Geometry check sheet. Reference: drawing and pictorial views, mm from the part's lowest x, y, z. Coordinates: 2 decimals unless noted, no trailing zeros. Loops run counter-clockwise (first coordinate to the right, second up) from the corner with the lowest first, then second, coordinate; pieces in that order, holes last.
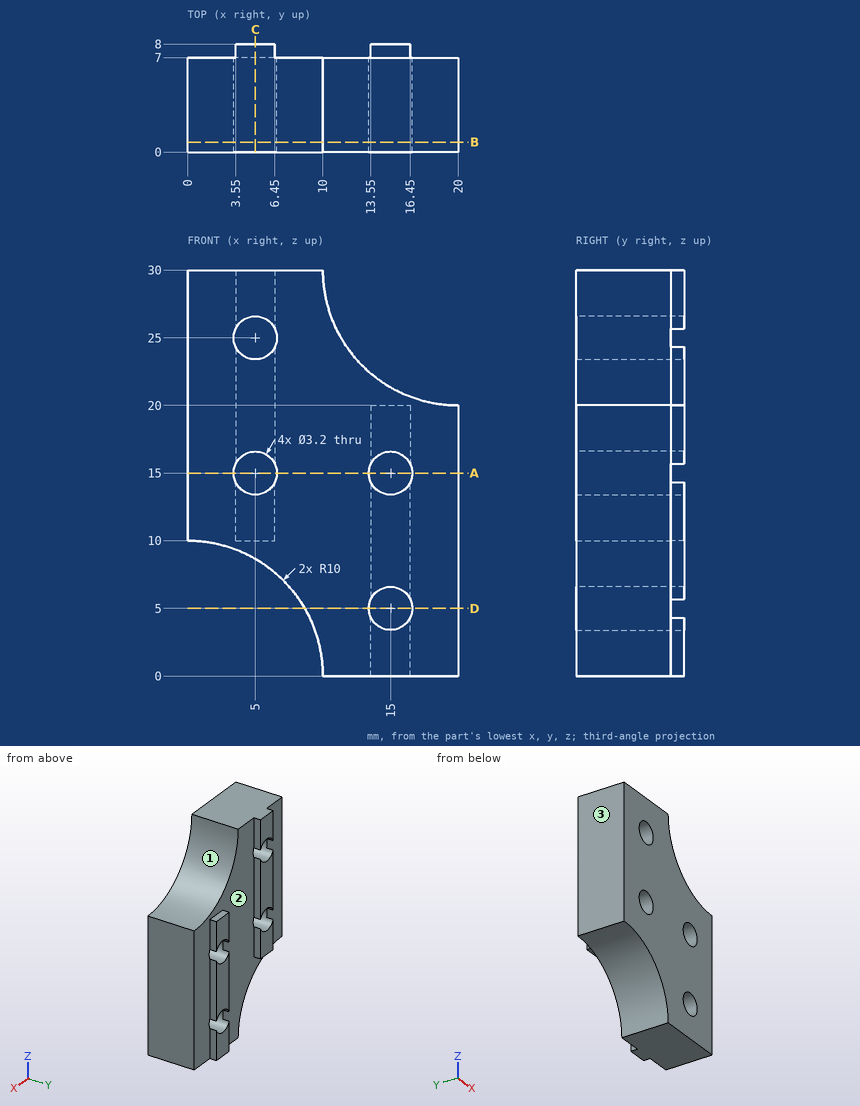
1) Depth check by flat-ended pin: pin 1 (0.8 mm diameter, centred on y = 7.5, z = 12.5, fed in from -X); pin 2 (0.8 mm diameter, centred on x = 5.5, y = 7.5, fed in from -Z); pin 3 (0.8 mm diameter, centred on y = 7.5, z = 17, fed in from +X). Enter the tip coordinate at first touch or a pass-through.
Data:
pin 1: stops at x = 3.55
pin 2: stops at z = 10
pin 3: stops at x = 16.45
2) Mould release check, pull along X, two halves, no side actions. Record for the marked faces 1, 2 and 3: +X half, -X half, draft (parallel to the pull), parting line (faces both ways), or undercut.
Data:
face 1: +X half
face 2: undercut
face 3: -X half
3) Section check C-C on x = 5. Record the cut outline in (y, z), and give its area (3 significant figures).
Data:
outline: (0, 8.66) - (7, 8.66) - (7, 10) - (8, 10) - (8, 13.4) - (0, 13.4) - close; (0, 16.6) - (8, 16.6) - (8, 23.4) - (0, 23.4) - close; (0, 26.6) - (8, 26.6) - (8, 30) - (0, 30) - close
area: 118 mm2
4) Section check B-B on y = 0.75. Count the separate pieces of the cut face and the enclosed holes in it, and give its area (3 significant figures).
Data:
separate pieces: 1
enclosed holes: 4
area: 411 mm2
5) Section check D-D on z = 5. Record the cut outline in (x, y), and give its area (3 significant figures).
Data:
outline: (8.66, 0) - (13.4, 0) - (13.4, 7) - (8.66, 7) - close; (16.6, 0) - (20, 0) - (20, 7) - (16.6, 7) - close
area: 57.0 mm2
6) Section check A-A on z = 15. Record the cut outline in (x, y).
Data:
outline: (0, 0) - (3.4, 0) - (3.4, 7) - (0, 7) - close; (6.6, 0) - (13.4, 0) - (13.4, 7) - (6.6, 7) - close; (16.6, 0) - (20, 0) - (20, 7) - (16.6, 7) - close
7) Material ranges on probe 1 along X at (y, z) = (5, 15); probe 2 along Z at (x, y) = (15, 3); probe 3 along Z at (x, y) = (14, 6.5), recorded low to high.
Data:
probe 1: x = 0 to 3.4, 6.6 to 13.4, 16.6 to 20
probe 2: z = 0 to 3.4, 6.6 to 13.4, 16.6 to 21.34
probe 3: z = 0 to 3.75, 6.25 to 13.75, 16.25 to 22
